CAD build for the part. Positions are in the model's coordinates, mm. A direction names the side the tool comes from. Round coordinates to 2 decimals unless told otherwise and drop trailing zeros. Order: outer loops, then holes, each group sorted by start corner. A loop starts at its lowest first (then second) coordinate and runs counter-clockwise, first axis right, second up. Notation, with made-up numbers: (-23, 34) -> (13, 34) arc R8 cw to (13, 40) -> close; hole circle Ø8 at (84, 43). An arc over 180 degrees is marked (long way). Answer as CSV lines item,"result". Start each with the question number.
from build123d import *

# Parameters (mm, degrees)
SKETCH_1_W          = 40
SKETCH_1_H          = 48
EXTRUDE_1_DEPTH     = 3
CHAMFER_1_SIZE      = 12
SKETCH_2_R          = 2.95
SKETCH_2_W          = 13
SKETCH_2_H          = 10.5
CUT_EXTRUDE_1_DEPTH = 10
EXTRUDE_2_DEPTH     = 3
FILLET_1_R          = 2
CUT_EXTRUDE_3_DEPTH = 3
SKETCH_10_R         = 1.7
CUT_EXTRUDE_4_DEPTH = 3
SKETCH_12_R         = 1.7
SKETCH_12_R_2       = 2.95
EXTRUDE_4_DEPTH     = 3
FILLET_2_R          = 3
FILLET_3_R          = 13
FILLET_4_R          = 3
EXTRUDE_5_DEPTH     = 3
FILLET_5_R          = 2


with BuildPart() as part:
    # 草图1 → 凸台-拉伸1 (new body)
    with BuildSketch(Plane.XY):
        with Locations((20, 24)):
            Rectangle(SKETCH_1_W, SKETCH_1_H)
    extrude(amount=EXTRUDE_1_DEPTH)

    # 倒角1
    chamfer_1_edges = [part.edges().sort_by_distance(p)[0] for p in [
        (0, 48, 1.5),
        (40, 48, 1.5),
    ]]
    chamfer(chamfer_1_edges, length=CHAMFER_1_SIZE)

    # 草图2 → 切除-拉伸1 (cut)
    with BuildSketch(Plane(origin=(0, 0, 0), x_dir=(-1, 0, 0), z_dir=(0, 0, -1))):
        with Locations((-20, 29.5)):
            Circle(SKETCH_2_R)
        with BuildLine():
            Line((-6.676784368, 4.473797691), (-6.5, 42.5))
            Line((-6.5, 42.5), (0, 36))
            Line((0, 36), (0, 0))
            Line((0, 0), (-1.349561874, 1.722051065))
            ThreePointArc((-1.349561874, 1.722051065), (-2.686952607, 5.665410674), (-6.676784368, 4.473797691))
        make_face()
        with BuildLine():
            Line((-33.5, 42.5), (-40, 36))
            Line((-40, 36), (-40, 0))
            Line((-40, 0), (-38.650438126, 1.722051065))
            ThreePointArc((-38.650438126, 1.722051065), (-37.313047393, 5.665410674), (-33.323215632, 4.473797691))
            Line((-33.323215632, 4.473797691), (-33.5, 42.5))
        make_face()
        with Locations((-20, 10.25)):
            Rectangle(SKETCH_2_W, SKETCH_2_H)
    extrude(amount=-CUT_EXTRUDE_1_DEPTH, mode=Mode.SUBTRACT)

    # 草图6 → 凸台-拉伸2 (add)
    with BuildSketch(Plane.XY.offset(3)):
        Polygon((0, 0), (0, 15), (6.588392184, 23.486898846), (6.676784368, 4.473797691), (1.450726441, 4.473797691), (1.450726441, 0), align=None)
        Polygon((40, 15), (33.411607816, 23.486898846), (33.323215632, 4.473797691), (38.549273559, 4.473797691), (38.549273559, 0), (40, 0), align=None)
    extrude(amount=-EXTRUDE_2_DEPTH)

    # 圆角1
    fillet_1_edges = [part.edges().sort_by_distance(p)[0] for p in [
        (13.5, 15.5, 1.5),
        (13.5, 5, 1.5),
        (26.5, 5, 1.5),
        (26.5, 15.5, 1.5),
    ]]
    fillet(fillet_1_edges, radius=FILLET_1_R)

    # 草图7 → 切除-拉伸3 (cut)
    with BuildSketch(Plane.XY.offset(3)):
        with BuildLine():
            Line((14, 40), (14, 23.857322167))
            ThreePointArc((14, 23.857322167), (12, 21.857322167), (10, 23.857322167))
            Line((10, 23.857322167), (10, 40))
            ThreePointArc((10, 40), (12, 42), (14, 40))
        make_face()
        with BuildLine():
            Line((26, 40), (26, 23.857322167))
            ThreePointArc((26, 23.857322167), (28, 21.857322167), (30, 23.857322167))
            Line((30, 23.857322167), (30, 40))
            ThreePointArc((30, 40), (28, 42), (26, 40))
        make_face()
    extrude(amount=-CUT_EXTRUDE_3_DEPTH, mode=Mode.SUBTRACT)

    # 草图10 → 切除-拉伸4 (cut)
    with BuildSketch(Plane(origin=(0, 0, 0), x_dir=(-1, 0, 0), z_dir=(0, 0, -1))):
        with Locations((-4.063755404, 3)):
            Circle(SKETCH_10_R)
        with Locations((-36.5, 3)):
            Circle(SKETCH_10_R)
    extrude(amount=-CUT_EXTRUDE_4_DEPTH, mode=Mode.SUBTRACT)

    # 草图12 → 凸台-拉伸4 (add)
    with BuildSketch(Plane.XY.offset(3)):
        Polygon((33.5, 0), (33.5, -33.5), (48.5, -33.5), (56.986898846, -26.911607816), (76, -27), (81.5, -21.5), (81.5, -5.5), (76, 0), (56.986898846, -0.088392184), (48.5, 6.5), (40, 6.5), (40, 0), align=None)
        with Locations((36.5, -29.436244596)):
            Circle(SKETCH_12_R, mode=Mode.SUBTRACT)
        with BuildLine():
            ThreePointArc((40.5, -20), (39.085786438, -19.414213562), (38.5, -18))
            Line((38.5, -18), (38.5, -9))
            ThreePointArc((38.5, -9), (39.085786438, -7.585786438), (40.5, -7))
            Line((40.5, -7), (47, -7))
            ThreePointArc((47, -7), (48.414213562, -7.585786438), (49, -9))
            Line((49, -9), (49, -18))
            ThreePointArc((49, -18), (48.414213562, -19.414213562), (47, -20))
            Line((47, -20), (40.5, -20))
        make_face(mode=Mode.SUBTRACT)
        with BuildLine():
            ThreePointArc((73.5, -19.5), (75.5, -21.5), (73.5, -23.5))
            Line((73.5, -23.5), (57.357322167, -23.5))
            ThreePointArc((57.357322167, -23.5), (55.357322167, -21.5), (57.357322167, -19.5))
            Line((57.357322167, -19.5), (73.5, -19.5))
        make_face(mode=Mode.SUBTRACT)
        with Locations((63, -13.5)):
            Circle(SKETCH_12_R_2, mode=Mode.SUBTRACT)
        with BuildLine():
            ThreePointArc((57.357322167, -7.5), (55.357322167, -5.5), (57.357322167, -3.5))
            Line((57.357322167, -3.5), (73.5, -3.5))
            ThreePointArc((73.5, -3.5), (75.5, -5.5), (73.5, -7.5))
            Line((73.5, -7.5), (57.357322167, -7.5))
        make_face(mode=Mode.SUBTRACT)
    extrude(amount=-EXTRUDE_4_DEPTH)

    # 圆角2
    fillet_2_edges = [part.edges().sort_by_distance(p)[0] for p in [
        (33.5, -33.5, 1.5),
        (33.5, 0, 1.5),
        (0, 0, 1.5),
    ]]
    fillet(fillet_2_edges, radius=FILLET_2_R)

    # 圆角3
    # the kernel refuses this fillet: 13 mm, written as the material it adds along each edge
    with BuildSketch(Plane(origin=(40, 6.5, 3), x_dir=(0, 1, 0), z_dir=(0, 0, -1))) as fillet_3_piece_1:
        with BuildLine():
            CenterArc((12.400920193, 12.400920193), FILLET_3_R, 197.46185463, 55.076290741)
            Line((0, 8.5), (0, 0))
            Line((0, 0), (8.5, 0))
        make_face()
    extrude(amount=3)

    # 圆角4
    fillet_4_edges = [part.edges().sort_by_distance(p)[0] for p in [
        (33.411607816, 23.486898846, 1.5),
        (56.986898846, -0.088392184, 1.5),
    ]]
    fillet(fillet_4_edges, radius=FILLET_4_R)

    # 草图13 → 凸台-拉伸5 (add)
    # profile 1 of 2: a face of its own
    with BuildSketch(Plane.XY.offset(3)):
        Polygon((34.046638715, 22.66887787), (57.042815657, 0.076069922), (39.491091869, 6.043623433), align=None)
    # profile 2 of 2: a face of its own
    with BuildSketch(Plane.XY.offset(3)):
        Polygon((0.878679656, 0.878679656), (34.378679656, -32.621320344), (34.046638715, 0.878679656), align=None)
        Polygon((10.535533906, -3.121320344), (30.281807462, -22.8675939), (30.086088917, -3.121320344), align=None, mode=Mode.SUBTRACT)
    extrude(amount=-EXTRUDE_5_DEPTH)

    # 圆角5
    fillet_5_edges = [part.edges().sort_by_distance(p)[0] for p in [
        (30.086088917, -3.121320344, 1.5),
        (30.281807462, -22.8675939, 1.5),
        (10.535533906, -3.121320344, 1.5),
    ]]
    fillet(fillet_5_edges, radius=FILLET_5_R)


solid = part.part
Item 1: Band-saw the part on C-C, the plane y = -12.5. Give the cut face in (x, z).
Item 2: Mould opens along X. For faces 1 (the flat face through (45.384, 11.531, 1.521)), 2 (the flat face through (32, -1, 3)), 3 (the cylindrical face through (14.1, 14.93, 1.52)) say: released by +X, released by -X, zero draft, split by the parting line, or undercut.
Item 3: Band-saw the part on D-D, the plane y = 34. Give the cut face in (x, z).
Item 4: Band-saw the part on A-A, the plane x = 68.5. Give the cut face in (y, z).
Item 5: Probe line 1 (Y direction, x = 59.5, z = 0.9); line 2 (Y direction, x = 36.5, z = 1.4); line 3 (X direction, y = 4, z = 0.3). List the from-to ranges inside material, lowest first.
Item 6: Pin check, flat tips, straight feed: pin 1 (2 mm diameter, centred on x = 20, y = 27.5, fed in from -Z); pin 2 (1 mm diameter, centred on x = 72.5, z = 1, fed in from +Y); pin 3 (0.9 mm diameter, centred on y = 34.5, z = 1, fed in from +X); pin 4 (0.9 mm diameter, centred on x = 66.5, z = 1, fed in from -Y). Stop position of each tip, or through.
Item 7: Band-saw the part on B-B, the plane y = 12. Give the cut face in (x, z), and give its area (3 significant figures).
Item 8: Tool access for faces 4 (the cylindrical face through (75.5, -5.5, 1.5)), 5 (the flat face through (20, 48, 1)), 6 (the cylindrical face through (33.58, 23.53, 1.48)): list every direction of +Z, -Z, +X, -X, +Y, -Y with a clear straight run to the whole face (end or side of a thin tool).
Values:
1,outline,"(14.26, 0) -> (19.91, 0) -> (19.91, 3) -> (14.26, 3) -> close; (30.18, 0) -> (38.5, 0) -> (38.5, 3) -> (30.18, 3) -> close; (49, 0) -> (60.22, 0) -> (60.22, 3) -> (49, 3) -> close; (65.78, 0) -> (81.5, 0) -> (81.5, 3) -> (65.78, 3) -> close"
2,face 1,"released by +X"
2,face 2,"zero draft"
2,face 3,"undercut"
3,outline,"(6.54, 0) -> (10, 0) -> (10, 3) -> (6.54, 3) -> close; (14, 0) -> (26, 0) -> (26, 3) -> (14, 3) -> close; (30, 0) -> (33.46, 0) -> (33.46, 3) -> (30, 3) -> close"
4,outline,"(-26.97, 0) -> (-23.5, 0) -> (-23.5, 3) -> (-26.97, 3) -> close; (-19.5, 0) -> (-7.5, 0) -> (-7.5, 3) -> (-19.5, 3) -> close; (-3.5, 0) -> (-0.03, 0) -> (-0.03, 3) -> (-3.5, 3) -> close"
5,line 1,"-26.92 to -23.5, -19.5 to -7.5, -3.5 to -0.08"
5,line 2,"-33.5 to -31.14, -27.74 to 1.3, 4.7 to 20.26"
5,line 3,"0 to 2.69, 5.44 to 35.13, 37.87 to 53.05"
6,pin 1,"z = 0"
6,pin 2,"y = -0.01"
6,pin 3,"x = 33.46"
6,pin 4,"y = -26.96"
7,outline,"(0, 0) -> (13.5, 0) -> (13.5, 3) -> (0, 3) -> close; (26.5, 0) -> (44.91, 0) -> (44.91, 3) -> (26.5, 3) -> close"
7,area,"95.7 mm²"
8,face 4,"+Z, -Z"
8,face 5,"+Z, -Z, +X, -X, +Y"
8,face 6,"+Z, -Z, +X"
